Autodesk Inventor part; units mm, degrees
ref_plane "YZ Plane" through (0, 0, 0) normal (1, 0, 0) x (0, 1, 0)
ref_plane "XZ Plane" through (0, 0, 0) normal (0, 1, 0) x (-1, 0, 0)
ref_plane "XY Plane" through (0, 0, 0) normal (0, 0, 1) x (1, 0, 0)
sketch "スケッチ1" plane through (0, 0, 0) normal (0, 0, 1) x (1, 0, 0)
  circle A0 centre (11.8968, -42.422) radius 1.6
  circle A1 centre (7.5, -33.4405) radius 1.6
  circle A2 centre (3.1032, -24.4589) radius 1.6
  circle A3 centre (7.5, 10) radius 1.6
  circle A4 centre (7.5, 20) radius 1.6
  circle A5 centre (7.5, 30) radius 1.6
  line L0 (-6.9305, -21.0203) -> (8.4582, -52.4558)
  line L1 (8.4582, -52.4558) -> (21.9305, -45.8606)
  line L2 (15, 0) -> (15, 37.5)
  line L3 (15, 37.5) -> (0, 37.5)
  line L4 (0, 37.5) -> (0, 0)
  arc A6 (15, 0) -> (21.9305, -45.8606) centre (91.2366, -11.933) ccw
  line L5 (21.9305, -45.8606) -> (6.5418, -14.4252) construction
  arc A7 (-6.9305, -21.0203) -> (0, 0) centre (-35.3427, 0) ccw
  line L6 (6.5418, -14.4252) -> (-6.9305, -21.0203) construction
  dimension "d0" = 7.5
  dimension "d1" = 7.5
  dimension "d2" = 7.5
  dimension "d3" = 7.5
  dimension "d4" = 7.5
  dimension "d5" = 7.5
  dimension "d6" = 7.5
extrude "押し出し1" add sketch "スケッチ1" along normal blind 3
fillet "フィレット1" radius 2 6 edges at (21.9305, -45.8606, 1.5) (8.4582, -52.4558, 1.5) (-6.9305, -21.0203, 1.5) (0, 37.5, 1.5) (15, 37.5, 1.5) (15, 0, 1.5)
properties part number "オムニ_固定具寸法不明2" material "アルミニウム 6061"
Verification items for the finished model (mm, model axes). A direction names the side the tool comes from. Coordinates: 2 decimals unless noted, no trailing zeros. Loops run counter-clockwise (first coordinate to the right, second up) from the corner with the lowest first, then second, coordinate; pieces in that order, holes last. Notation, with made-up numbers: (21, 41.5) - (35, 41.5) arc R26 ccw to (35, 59.5) - close; hole circle Ø8 at (71, 51). An arc over 180 degrees is marked (long way). Return JSON: item names as keys, results as strings.
1. Tool access check on faces 4 (the flat face through (15, 18, 1)), 5 (the flat face through (15.136, -49.187, 1.479)), 6 (the flat face through (0, 18, 1)). Record the directions out of +Z, -Z, +X, -X, +Y, -Y that give a thin tool (end or side, any length) a straight path to the whole face; none if there is none.
Established:
{"face 4": "+Z, -Z, +X, +Y", "face 5": "+Z, -Z, +X, -Y", "face 6": "+Z, -Z, -X, +Y"}
2. Section check C-C, the plane z = 1.35. Count the separate pieces of the cut face and the enclosed holes in it, then the cut area to 3 significant figures.
Established:
{"separate pieces": "1", "enclosed holes": "6", "area": "1,370 mm2"}
3. Mould release check, pull along Y, two halves, no side actions. Record for faces 1 (the cylindrical face through (7.15, 11.56, 1.48)), 2 (the cylindrical face through (-6.6, -21, 1.5)), 3 (the cylindrical face through (0.6, 36.93, 1.52)): +Y half, -Y half, draft (parallel to the pull), parting line (faces both ways), or undercut.
Established:
{"face 1": "undercut", "face 2": "parting line", "face 3": "+Y half"}
4. Go/stop test with flat-tipped pins: pin 1 (2.5 mm diameter, centred on x = 7.5, y = 20, fed in from +Z); pin 2 (1.5 mm diameter, centred on y = -23, z = 0.5, fed in from +X); pin 3 (1.5 mm diameter, centred on y = 19, z = 2, fed in from -X). Record where each tip stops, or that it passes through.
Established:
{"pin 1": "passes through", "pin 2": "stops at x = 14.98", "pin 3": "stops at x = 0"}
5. Section check A-A, the plane y = 20. Record the boundary of the cut face in (x, z), then the cut area to 3 significant figures.
Established:
{"outline": "(0, 0) - (5.9, 0) - (5.9, 3) - (0, 3) - close; (9.1, 0) - (15, 0) - (15, 3) - (9.1, 3) - close", "area": "35.4 mm2"}
6. Thickness scan on L1, parallel to Y at x = 7.5, z = 1.5; L2, parallel to X at y = -25, z = 2.75; L3, parallel to X at y = 5, z = 2.8. Record the ranges inside material, lowest first.
Established:
{"L1": "y = -50.5 to -35.04, -31.84 to 8.4, 11.6 to 18.4, 21.6 to 28.4, 31.6 to 37.5", "L2": "x = -4.98 to 1.6, 4.61 to 15.19", "L3": "x = 0 to 15"}
7. Section check B-B, the plane x = 3.5. Record the boundary of the cut face in (y, z), then the cut area to 3 significant figures.
Established:
{"outline": "(-42.33, 0) - (-26.01, 0) - (-26.01, 3) - (-42.33, 3) - close; (-22.91, 0) - (37.5, 0) - (37.5, 3) - (-22.91, 3) - close", "area": "230 mm2"}
8. Section check D-D, the plane y = -40. Record the boundary of the cut face in (x, z).
Established:
{"outline": "(2.36, 0) - (19.36, 0) - (19.36, 3) - (2.36, 3) - close"}
